from build123d import *

# Parameters (mm, degrees)
SKETCH_1_W          = 68
SKETCH_1_H          = 50
SKETCH_1_R          = 3
EXTRUDE_1_DEPTH     = 6
SKETCH_3_W          = 68
SKETCH_3_H          = 6
EXTRUDE_2_DEPTH     = 50
CUT_EXTRUDE_1_REACH = 8
SKETCH_4_R          = 12.5
SKETCH_4_R_2        = 3.5


with BuildPart() as part:
    # 草图1 → 凸台-拉伸1 (new body)
    with BuildSketch(Plane(origin=(0, 0, 0), x_dir=(1, 0, 0), z_dir=(0, 1, 0))):
        with Locations((0, 25)):
            Rectangle(SKETCH_1_W, SKETCH_1_H)
        with Locations((-27.5, 35)):
            Circle(SKETCH_1_R, mode=Mode.SUBTRACT)
        with Locations((27.5, 35)):
            Circle(SKETCH_1_R, mode=Mode.SUBTRACT)
        with Locations((-27.5, 15)):
            Circle(SKETCH_1_R, mode=Mode.SUBTRACT)
        with Locations((27.5, 15)):
            Circle(SKETCH_1_R, mode=Mode.SUBTRACT)
    extrude(amount=EXTRUDE_1_DEPTH)

    # 草图3 → 凸台-拉伸2 (add)
    with BuildSketch(Plane(origin=(0, 6, 0), x_dir=(1, 0, 0), z_dir=(0, 1, 0))):
        with Locations((0, 47)):
            Rectangle(SKETCH_3_W, SKETCH_3_H)
    extrude(amount=-EXTRUDE_2_DEPTH)

    # 草图4 → 切除-拉伸1 (cut, up to next)
    with BuildSketch(Plane.XY.offset(-44), mode=Mode.PRIVATE) as cut_extrude_1_sk1:
        with Locations((0, -18)):
            Circle(SKETCH_4_R)
    cut_extrude_1_tool1 = extrude(cut_extrude_1_sk1.sketch, amount=-CUT_EXTRUDE_1_REACH, mode=Mode.PRIVATE) & part.part
    add(cut_extrude_1_tool1.solids().sort_by_distance((0, -18, -44))[0], mode=Mode.SUBTRACT)
    # 草图4 → 切除-拉伸1 (cut, up to next)
    with BuildSketch(Plane.XY.offset(-44), mode=Mode.PRIVATE) as cut_extrude_1_sk2:
        with Locations((28, -18)):
            Circle(SKETCH_4_R_2)
    cut_extrude_1_tool2 = extrude(cut_extrude_1_sk2.sketch, amount=-CUT_EXTRUDE_1_REACH, mode=Mode.PRIVATE) & part.part
    add(cut_extrude_1_tool2.solids().sort_by_distance((28, -18, -44))[0], mode=Mode.SUBTRACT)
    # 草图4 → 切除-拉伸1 (cut, up to next)
    with BuildSketch(Plane.XY.offset(-44), mode=Mode.PRIVATE) as cut_extrude_1_sk3:
        with Locations((-28, -18)):
            Circle(SKETCH_4_R_2)
    cut_extrude_1_tool3 = extrude(cut_extrude_1_sk3.sketch, amount=-CUT_EXTRUDE_1_REACH, mode=Mode.PRIVATE) & part.part
    add(cut_extrude_1_tool3.solids().sort_by_distance((-28, -18, -44))[0], mode=Mode.SUBTRACT)


solid = part.part
The listing builds one solid part. Answer for the finished solid, in the listing's coordinates (mm). A direction names the side the tool comes from. Give positions to 0.01 mm unless a question says otherwise; leave off trailing zeros. Write each loop counter-clockwise with the first axis right and the second up, starting at its lowest first coordinate (ties: lowest second). Pieces come first, ordered by that corner, then holes.
Item 1: Section A-A, the plane y = -18 is taken. Write down the section's boundary in (x, z), plus the area to 3 significant figures.
Item 2: Find the intervals of material crossed by line 1 along X through (y, z) = (2, -35); line 2 along Z through (x, y) = (27.5, 4.6); line 3 along X through (y, z) = (-16.5, -48), in increasing order.
Item 3: Section C-C, the plane x = -27.5 is taken. Write down the section's boundary in (y, z), plus the area to 3 significant figures.
Item 4: Section B-B, the plane z = -35 is taken. Write down the section's boundary in (x, y).
Item 5: Section D-D, the plane x = 0 is taken. Write down the section's boundary in (y, z), plus the area to 3 significant figures.
Item 6: Flat-ended cylindrical pins translate along their axes: P1, Ø10, axis at x = -26.5, y = -32.5, coming from the +Z side; P2, Ø1.5, axis at y = -15.5, z = -41.5, coming from the -X side; P3, Ø13, axis at x = -14.5, z = -12.5, coming from the -Y side. Find the tip coordinate at first contact, or state that the pin passes through.
Item 7: Which of the six approach directions +Z, -Z, +X, -X, +Y, -Y give full straight-line access (tool end or side, diameter ignored) to faces 1 (the cylindrical face through (-26.12, -15.05, -46.96)), 2 (the flat face through (0, -31, -44))?
Item 8: Determine the mould class of faces 3 (the flat face through (0, 3, 0)), 4 (the flat face through (0, 6, -25)), 5 (the cylindrical face through (25.29, 2.96, -37.03)) for opening direction Z: released by +Z, released by -Z, zero draft, split by the parting line, or undercut.
Completed:
1. outline: (-34, -50) - (-31.5, -50) - (-31.5, -44) - (-34, -44) - close; (-24.5, -50) - (-12.5, -50) - (-12.5, -44) - (-24.5, -44) - close; (12.5, -50) - (24.5, -50) - (24.5, -44) - (12.5, -44) - close; (31.5, -50) - (34, -50) - (34, -44) - (31.5, -44) - close
1. area: 174 mm2
2. line 1: x = -34 to -30.5, -24.5 to 24.5, 30.5 to 34
2. line 2: z = -50 to -38, -32 to -18, -12 to 0
2. line 3: x = -34 to -31.16, -24.84 to -12.41, 12.41 to 24.84, 31.16 to 34
3. outline: (-44, -50) - (-21.46, -50) - (-21.46, -44) - (-44, -44) - close; (-14.54, -50) - (6, -50) - (6, -38) - (0, -38) - (0, -44) - (-14.54, -44) - close; (0, -32) - (6, -32) - (6, -18) - (0, -18) - close; (0, -12) - (6, -12) - (6, 0) - (0, 0) - close
3. area: 450 mm2
4. outline: (-34, 0) - (-30.5, 0) - (-30.5, 6) - (-34, 6) - close; (-24.5, 0) - (24.5, 0) - (24.5, 6) - (-24.5, 6) - close; (30.5, 0) - (34, 0) - (34, 6) - (30.5, 6) - close
5. outline: (-44, -50) - (-30.5, -50) - (-30.5, -44) - (-44, -44) - close; (-5.5, -50) - (6, -50) - (6, 0) - (0, 0) - (0, -44) - (-5.5, -44) - close
5. area: 414 mm2
6. P1: stops at z = -44
6. P2: passes through
6. P3: stops at y = 0
7. face 1: +Z, -Z
7. face 2: +Z, +X, -X, -Y
8. face 3: released by +Z
8. face 4: zero draft
8. face 5: undercut
